For this review, use the dimensioned drawing (mm, ordinates from the lowest corner) and the shaded views. A direction names the side the tool comes from. Coordinates: 2 decimals unless noted, no trailing zeros. Loops run counter-clockwise (first coordinate to the right, second up) from the corner with the lowest first, then second, coordinate; pieces in that order, holes last. Notation, with made-up numbers: (56, 37.25) - (93, 37.25) arc R27 cw to (93, 59.25) - close; hole circle Ø9 at (-11, 20). An arc over 180 degrees is marked (long way). Answer in a Markdown table with one row per item. Add a question column.
(1) Clearance check with flat-ended pins moving along their axes: pin 1 (1.5 mm diameter, centred on x = 20.5, y = 11.5, fed in from +Z); pin 2 (1 mm diameter, centred on x = 41, z = 13, fed in from -Y); pin 3 (11 mm diameter, centred on x = 34, z = 12.5, fed in from +Y). State where each tip first meets the part, or that it passes through.
(2) We need section A-A, the plane z = 16. Write out the cut boundary in (x, y), plus the area to 3 significant figures.
(3) We need section D-D, the plane y = 2.75. Write out the cut boundary in (x, z) (1 decimal).
(4) The part is to be moulded in two halves that separate along Z. For the marked faces 1, 2, 3 and 4, say which applies: released by +Z, released by -Z, zero draft, split by the parting line, or undercut.
(5) To check wall thickness, follow L1, parallel to X at y = 14.5, z = 2; L2, parallel to Y at x = 35, z = 19; L3, parallel to Z at x = 20.5, y = 7.5 (1 decimal). State the ranges of each line that lie inside material, in increasing order. Write a range as [from, to].
(6) We need section B-B, the plane x = 2.8. Write out the cut boundary in (y, z).
(7) We need section C-C, the plane y = 11. Write out the cut boundary in (x, z).
(8) For the marked faces 5, 6, 7 and 8, list the 3-axis set-ups (+Z, -Z, +X, -X, +Y, -Y) from which the entire face can be reached by the end or side of a thin tool; tool diameter is ignored.
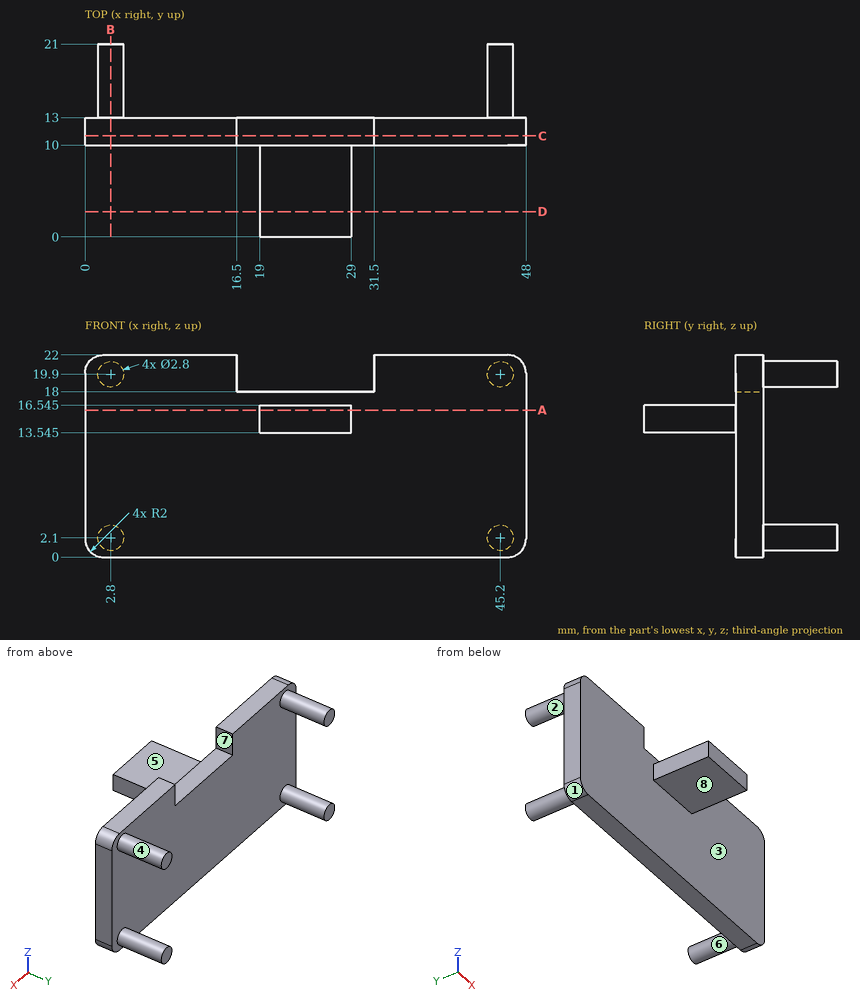
Responses:
| question | item | result |
|---|---|---|
| 1 | pin 1 | stops at z = 18 |
| 1 | pin 2 | stops at y = 10 |
| 1 | pin 3 | stops at y = 13 |
| 2 | outline | (0, 10) - (19, 10) - (19, 0) - (29, 0) - (29, 10) - (48, 10) - (48, 13) - (0, 13) - close |
| 2 | area | 244 mm2 |
| 3 | outline | (19, 13.5) - (29, 13.5) - (29, 16.5) - (19, 16.5) - close |
| 4 | face 1 | released by -Z |
| 4 | face 2 | undercut |
| 4 | face 3 | zero draft |
| 4 | face 4 | undercut |
| 5 | L1 | x = [1.4, 4.2], [43.8, 46.6] |
| 5 | L2 | y = [10, 13] |
| 5 | L3 | z = [13.5, 16.5] |
| 6 | outline | (10, 0) - (13, 0) - (13, 0.7) - (21, 0.7) - (21, 3.5) - (13, 3.5) - (13, 18.5) - (21, 18.5) - (21, 21.3) - (13, 21.3) - (13, 22) - (10, 22) - close |
| 7 | outline | (0, 2) arc R2 ccw to (2, 0) - (46, 0) arc R2 ccw to (48, 2) - (48, 20) arc R2 ccw to (46, 22) - (31.5, 22) - (31.5, 18) - (16.5, 18) - (16.5, 22) - (2, 22) arc R2 ccw to (0, 20) - close |
| 8 | face 5 | +Z, +X, -X, -Y |
| 8 | face 6 | +Y |
| 8 | face 7 | +Z, +Y, -Y |
| 8 | face 8 | -Z, +X, -X, -Y |
